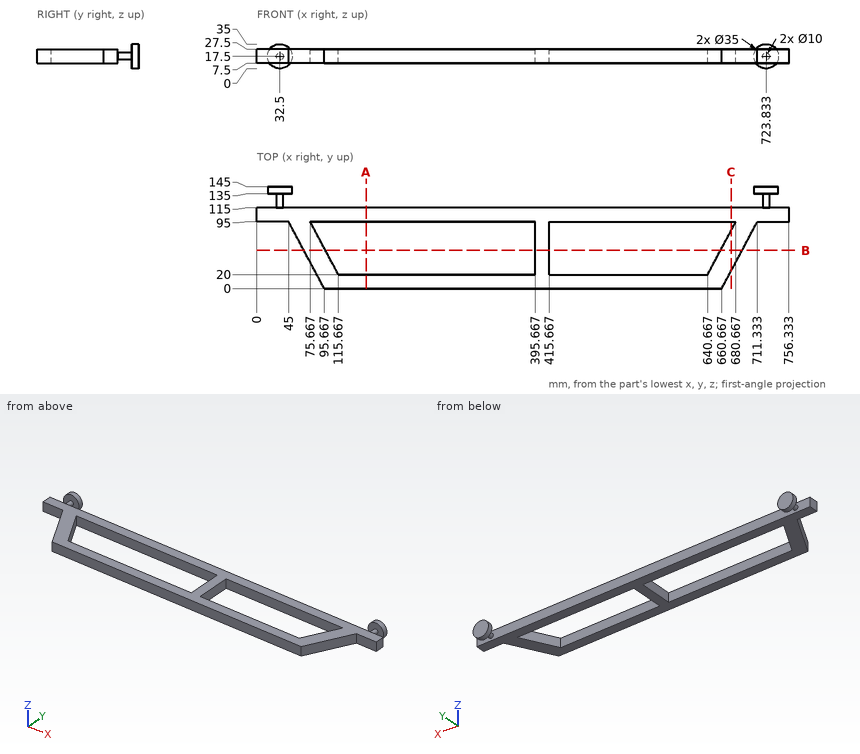
For this review, use the dimensioned drawing (mm, ordinates from the lowest corner) and the shaded views. Coordinates: 2 decimals unless noted, no trailing zeros. Loops run counter-clockwise (first coordinate to the right, second up) from the corner with the lowest first, then second, coordinate; pieces in that order, holes last. Notation, with made-up numbers: (63, -7.5) -> (117, -7.5) arc R22 ccw to (117, 9.5) -> close; hole circle Ø11 at (35.5, -10). An arc over 180 degrees is marked (long way). Use a Markdown table: item, result. Add a question column.
1. Add section A-A on x = 155. Write out the cut boundary in (y, z), plus the area to 3 significant figures.
2. Add section B-B on y = 54.5. Write out the cut boundary in (x, z), plus the area to 3 significant figures.
3. To check wall thickness, follow line 1 (Y direction, x = 269, z = 8.5); line 2 (X direction, y = 79, z = 23) (1 decimal); line 3 (Z direction, x = 605, y = 99.5). State the ranges of each line that lie inside material, in increasing order.
4. Add section C-C on x = 674. Write out the cut boundary in (y, z), plus the area to 3 significant figures.
5. Clearance check with flat-ended pins moving along their axes: pin 1 Ø10 at (y, z) = (66, 27) entering from -X; pin 2 Ø3 at (y, z) = (30, 25.5) entering from +X; pin 3 Ø10 at (y, z) = (47, 21.5) entering from -X. State where each tip first meets the part, or that it passes through.
Returned:
| question | item | result |
|---|---|---|
| 1 | outline | (0, 7.5) -> (20, 7.5) -> (20, 27.5) -> (0, 27.5) -> close; (95, 7.5) -> (115, 7.5) -> (115, 27.5) -> (95, 27.5) -> close |
| 1 | area | 800 mm² |
| 2 | outline | (66.6, 7.5) -> (97.27, 7.5) -> (97.27, 27.5) -> (66.6, 27.5) -> close; (395.67, 7.5) -> (415.67, 7.5) -> (415.67, 27.5) -> (395.67, 27.5) -> close; (659.07, 7.5) -> (689.73, 7.5) -> (689.73, 27.5) -> (659.07, 27.5) -> close |
| 2 | area | 1,630 mm² |
| 3 | line 1 | y = 0 to 20, 95 to 115 |
| 3 | line 2 | x = 53.5 to 84.2, 395.7 to 415.7, 672.1 to 702.8 |
| 3 | line 3 | z = 7.5 to 27.5 |
| 4 | outline | (25, 7.5) -> (82.5, 7.5) -> (82.5, 27.5) -> (25, 27.5) -> close; (95, 7.5) -> (115, 7.5) -> (115, 27.5) -> (95, 27.5) -> close |
| 4 | area | 1,550 mm² |
| 5 | pin 1 | stops at x = 57.8 |
| 5 | pin 2 | stops at x = 677.47 |
| 5 | pin 3 | stops at x = 67.93 |
